from build123d import *

# Parameters (mm, degrees)
F0_W     = 30
F0_H     = 50
F0_R     = 1.5
F1_DEPTH = 4
F2_W     = 18
F2_H     = 24
F3_DEPTH = 10
F4_W     = 18
F4_H     = 6
F5_DEPTH = 14


with BuildPart() as f1:
    # F0 (on Top) → F1 (new body)
    with BuildSketch(Plane.XY):
        Rectangle(F0_W, F0_H)
        with Locations((-10, -20)):
            Circle(F0_R, mode=Mode.SUBTRACT)
        with Locations((10, -20)):
            Circle(F0_R, mode=Mode.SUBTRACT)
        with Locations((-10, 20)):
            Circle(F0_R, mode=Mode.SUBTRACT)
        with Locations((10, 20)):
            Circle(F0_R, mode=Mode.SUBTRACT)
    extrude(amount=F1_DEPTH)

    # F2 (on face) → F3 (join)
    with BuildSketch(Plane(origin=(0, 0, 0), x_dir=(1, 0, 0), z_dir=(0, 0, -1))):
        Rectangle(F2_W, F2_H)
    extrude(amount=F3_DEPTH)

    # F4 (on face) → F5 (cut)
    with BuildSketch(Plane.YZ.offset(9)):
        with Locations((0, -5)):
            Rectangle(F4_W, F4_H)
    extrude(amount=-F5_DEPTH, mode=Mode.SUBTRACT)


solid = f1.part
The model under review builds one solid part; all positions refer to its coordinate system, in mm. A direction names the side the tool comes from. Round coordinates to 2 decimals unless told otherwise and drop trailing zeros. Write each loop counter-clockwise with the first axis right and the second up, starting at its lowest first coordinate (ties: lowest second). Pieces come first, ordered by that corner, then holes. Notation, with made-up numbers: M 36,83 L 64,83 A25 cw 64,101 Z; hole C 38,14 d6. An arc over 180 degrees is marked long. Answer as CSV lines item,"result". Start each with the question number.
Q1. Consider section C-C, the plane x = -10. Give the boundary of the cut face in (y, z), then the cut area to 3 significant figures.
Q2. Consider section B-B, the plane z = 2.25. Give the boundary of the cut face in (x, y).
Q3. Tool access review of faces 1 (the face through (-9, 0, -5)), 2 (the face through (2, 0, -2)), 3 (the face through (9, 0.2, -1.6)), 4 (the face through (0, 12, -5)), 5 (the face through (0, -12, -5)): name each direction out of +Z, -Z, +X, -X, +Y, -Y from which nothing blocks a thin tool from reaching the whole face with its end or side.
Q4. Consider section D-D, the plane y = -1.5. Give the boundary of the cut face in (x, z).
Q5. Consider section A-A, the plane y = 20. Give the boundary of the cut face in (x, z), then the cut area to 3 significant figures.
Q6. The part is to be moulded in two halves that separate along Y. For faces 6 (the face through (-5, 0, -5)), 7 (the face through (0, 0, 4)), 8 (the face through (0, -25, 2)), say which applies: +Y half, -Y half, draft (parallel to the pull), parting line (faces both ways), or undercut.
Q7. Wall thickness on line 1 along Y through (x, z) = (10, 2.6); line 2 along Z through (x, y) = (-1, -8); line 3 along Y through (x, z) = (-2, -2.5): over which ranges is each line inside the solid? List them lowest first.
Q8. Clearance check with flat-ended pins moving along their axes: P1, Ø5, axis at x = 0, z = -6.5, coming from the -Y side; P2, Ø5, axis at y = 4.5, z = -4.5, coming from the -X side; P3, Ø1.8, axis at x = 2, z = -5, coming from the +Y side. State where each tip first meets the part, or that it passes through.
Result set:
1,outline,"M -25,0 L -21.5,0 L -21.5,4 L -25,4 Z; M -18.5,0 L 18.5,0 L 18.5,4 L -18.5,4 Z; M 21.5,0 L 25,0 L 25,4 L 21.5,4 Z"
1,area,"176 mm²"
2,outline,"M -15,-25 L 15,-25 L 15,25 L -15,25 Z; hole C -10,-20 d3; hole C -10,20 d3; hole C 10,-20 d3; hole C 10,20 d3"
3,face 1,"-Z, -X, +Y, -Y"
3,face 2,"+X"
3,face 3,"-Z, +X, +Y, -Y"
3,face 4,"-Z, +X, -X, +Y"
3,face 5,"-Z, +X, -X, -Y"
4,outline,"M -15,0 L -9,0 L -9,-10 L 9,-10 L 9,-8 L -5,-8 L -5,-2 L 9,-2 L 9,0 L 15,0 L 15,4 L -15,4 Z"
5,outline,"M -15,0 L -11.5,0 L -11.5,4 L -15,4 Z; M -8.5,0 L 8.5,0 L 8.5,4 L -8.5,4 Z; M 11.5,0 L 15,0 L 15,4 L 11.5,4 Z"
5,area,"96.0 mm²"
6,face 6,"undercut"
6,face 7,"draft"
6,face 8,"-Y half"
7,line 1,"y = -25 to -21.5, -18.5 to 18.5, 21.5 to 25"
7,line 2,"z = -10 to -8, -2 to 4"
7,line 3,"y = -12 to -9, 9 to 12"
8,P1,"stops at y = -12"
8,P2,"stops at x = -9"
8,P3,"stops at y = 12"
